The listing builds one solid part. Answer for the finished solid, in the listing's coordinates (mm). A direction names the side the tool comes from. Give positions to 0.01 mm unless a question says otherwise; leave off trailing zeros. Order: outer loops, then holes, each group sorted by start corner. A loop starts at its lowest first (then second) coordinate and runs counter-clockwise, first axis right, second up. Notation, with made-up numbers: (26, -30.5) - (44, -30.5) arc R24 ccw to (44, 0.5) - close; hole circle Ø4 at (-1.75, 57.25). An arc over 180 degrees is marked (long way). Answer as a JSON object with one key per item and string values. Group by question number.
Q1. For faces 5 (the face through (-2.96, 2.96, 1.48)), 6 (the face through (-0.46, -2.32, 7.52)), 7 (the face through (2.443, -5.167, 1.479)), 8 (the face through (2.341, -0.466, 7.521)), 9 (the face through (5.167, 2.443, 1.479)), determine the directions among +Z, -Z, +X, -X, +Y, -Y from which every point of the face is accessible in a straight line to the end or side of a thin tool.
Q2. Given pin 1 (1.5 mm diameter, centred on x = 2, y = -1, fed in from +Z); pin 2 (1.5 mm diameter, centred on x = -2, y = 1.5, fed in from +Z); pin 3 (2.5 mm diameter, centred on x = 0, y = 0, fed in from +Z), each flat-ended and moving along its own axis, determine where each tip first touches the part or whether it passes through.
Q3. Consider line 1 (Y direction, x = 0, z = 5.75); line 2 (Z direction, x = 1.25, y = -2.5). Determine where each line is inside the solid, lowest interval first.
Q4. A cutting plane is placed at C-C, the plane z = 4. Give the vertices of the cut face in (x, y), and give its area (3 significant figures).
Q5. The mould has two halves that part along Y. Classify faces 1 (the face through (-2.443, 5.167, 1.479)), 2 (the face through (2, 1, 9)), 3 (the face through (-1.926, -5.381, 1.479)), 4 (the face through (-5.692, 0.269, 1.479)): released by +Y, released by -Y, zero draft, split by the parting line, or undercut.
Q6. A cutting plane is placed at B-B, the plane x = 4.5. Give the vertices of the cut face in (y, z).
Q7. A cutting plane is placed at A-A, the plane z = 6.5. Give the vertices of the cut face in (x, y).
from build123d import *

# Parameters (mm, degrees)
SALIENTE_EXTRUIR1_DEPTH = 3
CROQUIS2_R              = 3.25
SALIENTE_EXTRUIR2_DEPTH = 3
CROQUIS3_R              = 3.25
SALIENTE_EXTRUIR3_DEPTH = 3
CORTAR_EXTRUIR2_DEPTH   = 3
CROQUIS6_R              = 1.5
CORTAR_EXTRUIR3_DEPTH   = 10


with BuildPart() as part:
    # Croquis1 → Saliente-Extruir1 (new body)
    with BuildSketch(Plane.XY):
        with BuildLine():
            ThreePointArc((3.41860772, 0.359899305), (4.198868033, -0.004516375), (5.060021066, 0))
            ThreePointArc((5.060021066, 0), (5.700122231, -0.2741037), (6.204306422, -0.754375124))
            ThreePointArc((6.204306422, -0.754375124), (6.129908003, -1.219314513), (6.020718578, -1.67733354))
            ThreePointArc((6.020718578, -1.67733354), (5.371121207, -1.928103542), (4.674849897, -1.93638623))
            ThreePointArc((4.674849897, -1.93638623), (3.880976577, -1.602664645), (3.020654201, -1.640748138))
            ThreePointArc((3.020654201, -1.640748138), (2.858176792, -1.909772676), (2.67180794, -2.162833462))
            ThreePointArc((2.67180794, -2.162833462), (2.9658545, -2.972241619), (3.577975209, -3.577975209))
            ThreePointArc((3.577975209, -3.577975209), (3.836774498, -4.224415668), (3.853683377, -4.920530909))
            ThreePointArc((3.853683377, -4.920530909), (3.472313956, -5.196685077), (3.071237014, -5.443344854))
            ThreePointArc((3.071237014, -5.443344854), (2.434581138, -5.161331317), (1.93638623, -4.674849897))
            ThreePointArc((1.93638623, -4.674849897), (1.611009817, -3.877519894), (0.975740935, -3.296109203))
            ThreePointArc((0.975740935, -3.296109203), (0.670622982, -3.371449401), (0.359899305, -3.41860772))
            ThreePointArc((0.359899305, -3.41860772), (-0.004516375, -4.198868033), (0, -5.060021066))
            ThreePointArc((0, -5.060021066), (-0.2741037, -5.700122231), (-0.754375124, -6.204306422))
            ThreePointArc((-0.754375124, -6.204306422), (-1.219314513, -6.129908003), (-1.67733354, -6.020718578))
            ThreePointArc((-1.67733354, -6.020718578), (-1.928103542, -5.371121207), (-1.93638623, -4.674849897))
            ThreePointArc((-1.93638623, -4.674849897), (-1.602664645, -3.880976577), (-1.640748138, -3.020654201))
            ThreePointArc((-1.640748138, -3.020654201), (-1.909772676, -2.858176792), (-2.162833462, -2.67180794))
            ThreePointArc((-2.162833462, -2.67180794), (-2.972241619, -2.9658545), (-3.577975209, -3.577975209))
            ThreePointArc((-3.577975209, -3.577975209), (-4.224415668, -3.836774498), (-4.920530909, -3.853683377))
            ThreePointArc((-4.920530909, -3.853683377), (-5.196685077, -3.472313956), (-5.443344854, -3.071237014))
            ThreePointArc((-5.443344854, -3.071237014), (-5.161331317, -2.434581138), (-4.674849897, -1.93638623))
            ThreePointArc((-4.674849897, -1.93638623), (-3.877519894, -1.611009817), (-3.296109203, -0.975740935))
            ThreePointArc((-3.296109203, -0.975740935), (-3.371449401, -0.670622982), (-3.41860772, -0.359899305))
            ThreePointArc((-3.41860772, -0.359899305), (-4.198868033, 0.004516375), (-5.060021066, 0))
            ThreePointArc((-5.060021066, 0), (-5.700122231, 0.2741037), (-6.204306422, 0.754375124))
            ThreePointArc((-6.204306422, 0.754375124), (-6.129908003, 1.219314513), (-6.020718578, 1.67733354))
            ThreePointArc((-6.020718578, 1.67733354), (-5.371121207, 1.928103542), (-4.674849897, 1.93638623))
            ThreePointArc((-4.674849897, 1.93638623), (-3.880976577, 1.602664645), (-3.020654201, 1.640748138))
            ThreePointArc((-3.020654201, 1.640748138), (-2.858176792, 1.909772676), (-2.67180794, 2.162833462))
            ThreePointArc((-2.67180794, 2.162833462), (-2.9658545, 2.972241619), (-3.577975209, 3.577975209))
            ThreePointArc((-3.577975209, 3.577975209), (-3.836774498, 4.224415668), (-3.853683377, 4.920530909))
            ThreePointArc((-3.853683377, 4.920530909), (-3.472313956, 5.196685077), (-3.071237014, 5.443344854))
            ThreePointArc((-3.071237014, 5.443344854), (-2.434581138, 5.161331317), (-1.93638623, 4.674849897))
            ThreePointArc((-1.93638623, 4.674849897), (-1.611009817, 3.877519894), (-0.975740935, 3.296109203))
            ThreePointArc((-0.975740935, 3.296109203), (-0.670622982, 3.371449401), (-0.359899305, 3.41860772))
            ThreePointArc((-0.359899305, 3.41860772), (0.004516375, 4.198868033), (0, 5.060021066))
            ThreePointArc((0, 5.060021066), (0.2741037, 5.700122231), (0.754375124, 6.204306422))
            ThreePointArc((0.754375124, 6.204306422), (1.219314513, 6.129908003), (1.67733354, 6.020718578))
            ThreePointArc((1.67733354, 6.020718578), (1.928103542, 5.371121207), (1.93638623, 4.674849897))
            ThreePointArc((1.93638623, 4.674849897), (1.602664645, 3.880976577), (1.640748138, 3.020654201))
            ThreePointArc((1.640748138, 3.020654201), (1.909772676, 2.858176792), (2.162833462, 2.67180794))
            ThreePointArc((2.162833462, 2.67180794), (2.972241619, 2.9658545), (3.577975209, 3.577975209))
            ThreePointArc((3.577975209, 3.577975209), (4.224415668, 3.836774498), (4.920530909, 3.853683377))
            ThreePointArc((4.920530909, 3.853683377), (5.196685077, 3.472313956), (5.443344854, 3.071237014))
            ThreePointArc((5.443344854, 3.071237014), (5.161331317, 2.434581138), (4.674849897, 1.93638623))
            ThreePointArc((4.674849897, 1.93638623), (3.877519894, 1.611009817), (3.296109203, 0.975740935))
            ThreePointArc((3.296109203, 0.975740935), (3.371449401, 0.670622982), (3.41860772, 0.359899305))
        make_face()
    extrude(amount=SALIENTE_EXTRUIR1_DEPTH)

    # Croquis2 → Saliente-Extruir2 (add)
    with BuildSketch(Plane.XY.offset(3)):
        Circle(CROQUIS2_R)
    extrude(amount=SALIENTE_EXTRUIR2_DEPTH)

    # Croquis3 → Saliente-Extruir3 (add)
    with BuildSketch(Plane.XY.offset(6)):
        Circle(CROQUIS3_R)
    extrude(amount=SALIENTE_EXTRUIR3_DEPTH)

    # Croquis4 → Cortar-Extruir2 (cut)
    with BuildSketch(Plane.XY.offset(9)):
        with BuildLine():
            Line((0.292635483, 1.471177921), (1.219314513, 6.129908003))
            Line((1.219314513, 6.129908003), (-6.129908003, 1.219314513))
            Line((-6.129908003, 1.219314513), (-1.471177921, 0.292635483))
            ThreePointArc((-1.471177921, 0.292635483), (-1.247204418, -0.83335535), (-0.292635483, -1.471177921))
            Line((-0.292635483, -1.471177921), (-1.219314513, -6.129908003))
            Line((-1.219314513, -6.129908003), (6.129908003, -1.219314513))
            Line((6.129908003, -1.219314513), (1.471177921, -0.292635483))
            ThreePointArc((1.471177921, -0.292635483), (1.247204418, 0.83335535), (0.292635483, 1.471177921))
        make_face()
    extrude(amount=-CORTAR_EXTRUIR2_DEPTH, mode=Mode.SUBTRACT)

    # Croquis6 → Cortar-Extruir3 (cut)
    with BuildSketch(Plane.XY.offset(6)):
        Circle(CROQUIS6_R)
    extrude(amount=-CORTAR_EXTRUIR3_DEPTH, mode=Mode.SUBTRACT)


solid = part.part
Reply:
{
 "1": {"face 5": "+Z, -Z, -X", "face 6": "+Z, +X, -Y", "face 7": "+Z, -Z, -Y", "face 8": "+Z, -Y", "face 9": "+Z, -Z, +X"},
 "2": {"pin 1": "stops at z = 9", "pin 2": "stops at z = 6", "pin 3": "passes through"},
 "3": {"line 1": "y = -3.25 to -1.5, 1.5 to 3.25", "line 2": "z = 0 to 6"},
 "4": {"outline": "circle Ø6.5 at (0, 0); hole circle Ø3 at (0, 0)", "area": "26.1 mm^2"},
 "5": {"face 1": "released by +Y", "face 2": "zero draft", "face 3": "undercut", "face 4": "undercut"},
 "6": {"outline": "(-1.83, 0) - (-0.05, 0) - (-0.05, 3) - (-1.83, 3) - close; (1.9, 0) - (3.87, 0) - (3.87, 3) - (1.9, 3) - close"},
 "7": {"outline": "(-3.19, 0.63) arc R3.25 ccw to (-0.63, -3.19) - (-0.29, -1.47) arc R1.5 cw to (-1.47, 0.29) - close; (0.29, 1.47) arc R1.5 cw to (1.47, -0.29) - (3.19, -0.63) arc R3.25 ccw to (0.63, 3.19) - close"}
}
